Build history of the part. All positions in model axes, mm. Face numbers are marked on the shaded views. Round coordinates to 2 decimals unless told otherwise and drop trailing zeros. Write each loop counter-clockwise with the first axis right and the second up, starting at its lowest first coordinate (ties: lowest second). Pieces come first, ordered by that corner, then holes.
1) Saw through at A-A (y = 1.25). Write the cut outline in (x, z).
2) Wall check: probe 1 along Z at (x, y) = (-62, 0.9); probe 2 along Z at (x, y) = (-59.5, 1.75); probe 3 along Z at (x, y) = (-67.5, 0.3). Give the ranges that are in metal, low to high.
3) Flat gauge pin, fed straight in: pin 1 (2 mm diameter, centred on y = 3, z = -15.5, fed in from +X). Where does the tip first touch, or does it go through?
4) Pull direction Z, two halves, no side cores. Call the marked faces 1 and 2: +Z half, -Z half, draft (parallel to the pull), parting line (faces both ways), or undercut.
from build123d import *

# Parameters (mm, degrees)
SALIENTE_EXTRUIR1_DEPTH = 4
REDONDEO6_R             = 0.8


with BuildPart() as part:
    # Croquis1 → Saliente-Extruir1 (new body)
    with BuildSketch(Plane(origin=(0, 0, 0), x_dir=(1, 0, 0), z_dir=(0, 1, 0))):
        with BuildLine():
            ThreePointArc((-61.883639125, 14.575898233), (-67.780374095, 1.042618708), (-53.773153629, -3.61773673))
            ThreePointArc((-53.773153629, -3.61773673), (-63.274753441, 3.910149301), (-58.646815221, 15.11424029))
            ThreePointArc((-58.646815221, 15.11424029), (-60.82603012, 18.216941024), (-61.883639125, 14.575898233))
        make_face()
    extrude(amount=SALIENTE_EXTRUIR1_DEPTH)

    # Redondeo6
    # the kernel refuses this fillet: 0.8 mm, written as the material it takes off along each edge
    with BuildSketch(Plane(origin=(-53.533974817, 4, -6.444492505), x_dir=(0.17426350002173693, 0, 0.9846990568494387), z_dir=(0.9846990568494387, 0, -0.17426350002173693))) as redondeo6_piece_1:
        with BuildLine():
            CenterArc((10.065071469 + REDONDEO6_R, REDONDEO6_R), REDONDEO6_R, 180, 90)
            Line((10.065071469 + REDONDEO6_R, 0), (10.065071469, 0))
            Line((10.065071469, 0), (10.065071469, REDONDEO6_R))
        make_face()
    revolve(axis=Axis((-53.533974817, 4, -6.444492505), (0, -1, 0)), revolution_arc=170.903989059, mode=Mode.SUBTRACT)
    with BuildSketch(Plane(origin=(-58.646815221, 4, -5.11424029), x_dir=(-0.12889969509175428, 0, -0.9916576367906682), z_dir=(0.9916576367906682, 0, -0.12889969509175428))) as redondeo6_piece_2_section:
        with BuildLine():
            CenterArc((10 - REDONDEO6_R, -REDONDEO6_R), REDONDEO6_R, 0, 90)
            Line((10 - REDONDEO6_R, 0), (10, 0))
            Line((10, 0), (10, -REDONDEO6_R))
        make_face()
    redondeo6_piece_2 = revolve(axis=Axis((-58.646815221, 4, -5.11424029), (0, 1, 0)), revolution_arc=213.241351406, mode=Mode.PRIVATE)
    redondeo6_piece_2 = redondeo6_piece_2 - Plane(origin=(-60.481031052, 3.778290137, -16.142607032), x_dir=(0.8722614376655369, 0, 0.48903985968594704), z_dir=(0, -1, 0)) * Cylinder(2.102828064, 41, mode=Mode.PRIVATE)
    add(redondeo6_piece_2, mode=Mode.SUBTRACT)


solid = part.part
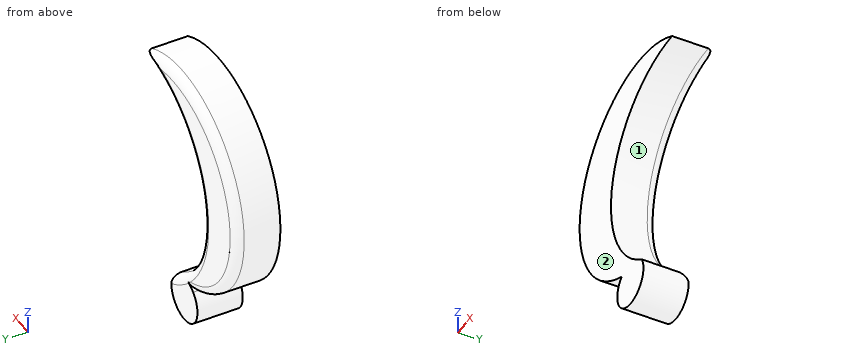
Evaluation:
1. outline: (-61.88, -14.58) arc R2.1 ccw (long way) to (-58.65, -15.11) arc R10.07 cw to (-53.77, 3.62) arc R10 ccw (long way) to start
2. probe 1: z = -17.6 to -14.69, -14.54 to -11.89, -1 to 4.31
2. probe 2: z = -18 to -14.55, 1.66 to 4.85
2. probe 3: z = -9.76 to -0.46
3. pin 1: stops at x = -58.38
4. face 1: undercut
4. face 2: draft
